The listing builds one solid part. Answer for the finished solid, in the listing's coordinates (mm). Coordinates: 2 decimals unless noted, no trailing zeros. Order: outer loops, then holes, each group sorted by start corner. A loop starts at its lowest first (then second) coordinate and runs counter-clockwise, first axis right, second up.
```python
from build123d import *

# Parameters (mm, degrees)
BOSS_EXTRUDE1_DEPTH = 0.04


with BuildPart() as part:
    # Sketch1 → Boss-Extrude1 (new body)
    with BuildSketch(Plane.XY):
        with BuildLine():
            Line((-1.570502823, 0.15738204), (-1.450502823, -0.00261796))
            Line((-1.450502823, -0.00261796), (8.549497177, -0.00261796))
            Line((8.549497177, -0.00261796), (9.189497177, 0.31738204))
            Line((9.189497177, 0.31738204), (10.289497177, 0.31738204))
            Line((10.289497177, 0.31738204), (10.319580052, 0.31738204))
            ThreePointArc((10.319580052, 0.31738204), (14.789486943, -0.056102846), (10.317408472, -0.40261796))
            Line((10.317408472, -0.40261796), (10.289497177, -0.40261796))
            Line((10.289497177, -0.40261796), (9.489497177, -0.40261796))
            Line((9.489497177, -0.40261796), (9.489497177, -4.90261796))
            Line((9.489497177, -4.90261796), (9.489497177, -4.917771037))
            ThreePointArc((9.489497177, -4.917771037), (9.339497177, -6.40261796), (9.189497177, -4.917771037))
            Line((9.189497177, -4.917771037), (9.189497177, -4.90261796))
            Line((9.189497177, -4.90261796), (9.189497177, -0.40261796))
            Line((9.189497177, -0.40261796), (8.549497177, -0.08261796))
            Line((8.549497177, -0.08261796), (-1.450502823, -0.08261796))
            Line((-1.450502823, -0.08261796), (-1.553035543, -0.24261796))
            Line((-1.553035543, -0.24261796), (-1.713035543, -0.24261796))
            Line((-1.713035543, -0.24261796), (-1.713035543, -4.74261796))
            Line((-1.713035543, -4.74261796), (-1.713035543, -4.757771037))
            ThreePointArc((-1.713035543, -4.757771037), (-1.863035543, -6.24261796), (-2.013035543, -4.757771037))
            Line((-2.013035543, -4.757771037), (-2.013035543, -4.74261796))
            Line((-2.013035543, -4.74261796), (-2.013035543, -0.24261796))
            Line((-2.013035543, -0.24261796), (-2.213035543, -0.24261796))
            Line((-2.213035543, -0.24261796), (-4.46302474, -4.139738514))
            Line((-4.46302474, -4.139738514), (-4.470603357, -4.152862955))
            ThreePointArc((-4.470603357, -4.152862955), (-5.342938887, -5.363770652), (-4.730431778, -4.002851195))
            Line((-4.730431778, -4.002851195), (-4.722853967, -3.98972604))
            Line((-4.722853967, -3.98972604), (-2.447853967, -0.049310453))
            Line((-2.447853967, -0.049310453), (-6.506560021, 2.29398458))
            Line((-6.506560021, 2.29398458), (-6.519672146, 2.301573339))
            ThreePointArc((-6.519672146, 2.301573339), (-7.730602208, 3.173881322), (-6.369682971, 2.56136874))
            Line((-6.369682971, 2.56136874), (-6.356560021, 2.553792202))
            Line((-6.356560021, 2.553792202), (-2.459445704, 0.303792202))
            Line((-2.459445704, 0.303792202), (-2.191269912, 0.15738204))
            Line((-2.191269912, 0.15738204), (-1.850502745, 0.15738204))
            Line((-1.850502745, 0.15738204), (-1.570502823, 0.15738204))
        make_face()
    extrude(amount=BOSS_EXTRUDE1_DEPTH)


solid = part.part
```
(1) Find section C-C (y = -1). Write down the section's boundary in (x, z).
(2) Find section B-B (x = -3). Write down the section's boundary in (y, z), and give its area (3 significant figures).
(3) This flat-tipped pin is pushed along its axis until it touches: pin 1 Ø4 at (x, y) = (-4.5, 1) entering from +Z. Where does it stop, or does it pass through?
(4) Find section D-D (x = 2.25). Write down the section's boundary in (y, z), and give its area (3 significant figures).
(5) Find section A-A (y = -4.5). Write down the section's boundary in (x, z), and give its area (3 significant figures).
Findings below:
1. outline: (-3, 0) - (-2.65, 0) - (-2.65, 0.04) - (-3, 0.04) - close; (-2.01, 0) - (-1.71, 0) - (-1.71, 0.04) - (-2.01, 0.04) - close; (9.19, 0) - (9.49, 0) - (9.49, 0.04) - (9.19, 0.04) - close; (10.5, 0) - (14.58, 0) - (14.58, 0.04) - (10.5, 0.04) - close
2. outline: (-1.61, 0) - (-1.01, 0) - (-1.01, 0.04) - (-1.61, 0.04) - close; (0.27, 0) - (0.62, 0) - (0.62, 0.04) - (0.27, 0.04) - close
2. area: 0.0379 mm2
3. pin 1: stops at z = 0.04
4. outline: (-0.08, 0) - (0, 0) - (0, 0.04) - (-0.08, 0.04) - close
4. area: 0.00320 mm2
5. outline: (-5.69, 0) - (-4.25, 0) - (-4.25, 0.04) - (-5.69, 0.04) - close; (-2.01, 0) - (-1.71, 0) - (-1.71, 0.04) - (-2.01, 0.04) - close; (9.19, 0) - (9.49, 0) - (9.49, 0.04) - (9.19, 0.04) - close
5. area: 0.0815 mm2
